Source: CAD feature listing. Evaluate the final solid. Frame: model axes, mm. A direction names the side the tool comes from. Coordinates: 2 decimals unless noted, no trailing zeros. Order: outer loops, then holes, each group sorted by start corner. A loop starts at its lowest first (then second) coordinate and runs counter-clockwise, first axis right, second up. Notation, with made-up numbers: (50.5, 60.25) - (78.5, 60.25) arc R24 cw to (78.5, 95.25) - close; hole circle Ø2 at (-31.5, 67). An arc over 180 degrees is marked (long way). One line per question, with ' | ' between items. Start each with the question number.
(1) Line query: line 1 along X through (y, z) = (7.5, 1.75); line 2 along X through (y, z) = (-4.5, 5.75); line 3 along Y through (x, z) = (-25.5, 6.5). Output: solid intervals per line, ascending.
(2) Contact query for flat-ended pins moving along their axis: P1, Ø4, axis at y = -67.5, z = 9.5, coming from the +X side; P2, Ø1.5, axis at y = -38.5, z = 6, coming from the -X side; P3, Ø1.2, axis at y = 19.5, z = 6.5, coming from the -X side. Output: stop coordinate, or through.
(3) Section B-B (x = -93.5). Return the cut outline in (y, z).
(4) Section C-C (x = -69.5). Return the cut outline in (y, z).
(5) Draft query along X for faces 5 (the flat face through (-25, -92.998, 6)), 6 (the cylindrical face through (73.76, 16.4, 11.01)), 7 (the flat face through (31, -8, 8)). Return one class per face: +X half, -X half, draft (parallel to the pull), parting line (faces both ways), or undercut.
(6) Access query for faces 1 (the flat face through (-90, 20, 6)), 2 (the flat face through (-44.33, -11, 8)), 3 (the flat face through (-72, -2, 6)), 4 (the flat face through (-53, 18.556, 8)). Directions: +Z, -Z, +X, -X, +Y, -Y. A direction counts if a zero-diameter tool reaches every point of the face in a straight line with its end or side. Return the directions, or none.
(7) Section A-A (z = 2). Return the cut outline in (x, y).
from build123d import *

# Parameters (mm, degrees)
BOSS_EXTRUDE1_DEPTH       = 12
SKETCH2_W                 = 25
SKETCH2_H                 = 26.555679241
CUT_EXTRUDE2_DEPTH        = 8
CUT_EXTRUDE8_START        = 4
SKETCH3_W                 = 3
SKETCH3_H                 = 36.555679241
CUT_EXTRUDE8_DEPTH        = 10
SKETCH5_W                 = 12
SKETCH5_H                 = 30.970366581
CUT_EXTRUDE10_DEPTH       = 18
LPATTERN1_COUNT           = 3
LPATTERN1_PITCH           = 42
LPATTERN2_COUNT           = 2
LPATTERN2_PITCH           = 42
CRVPATTERN1_START         = -70.397064899
CRVPATTERN1_OUTLINE_W     = 20.555679241
CRVPATTERN1_OUTLINE_H     = 8
CRVPATTERN1_DEPTH         = 37
CRVPATTERN1_2_DEPTH       = 12
CRVPATTERN1_START_2       = -58.397064899
CRVPATTERN1_3_OUTLINE_W   = 6
CRVPATTERN1_3_OUTLINE_H   = 8
CRVPATTERN1_3_DEPTH       = 25
CRVPATTERN1_START_3       = -53.397064899
CRVPATTERN1_4_OUTLINE_W   = 4
CRVPATTERN1_4_OUTLINE_H   = 8
CRVPATTERN1_4_OUTLINE_W_2 = 6
CRVPATTERN1_4_DEPTH       = 3
FILLET1_R                 = 10
FILLET2_R                 = 10
FILLET3_R                 = 10


# Read off the part's stored shape, not the designer's step: CrvPattern1
with BuildPart() as part:
    # Sketch1 → Boss-Extrude1 (new body)
    with BuildSketch(Plane.XY):
        Polygon((-111.658778955, 20), (77.777911134, 20), (59.936522952, -92.998049549), (-111.658778955, -92.998049549), align=None)
    extrude(amount=BOSS_EXTRUDE1_DEPTH)

    # Sketch2 → Cut-Extrude2 (cut)
    with BuildSketch(Plane.XY.offset(12)):
        with Locations((-6.829680892, 5.27783962)):
            Rectangle(SKETCH2_W, SKETCH2_H)
    cut_extrude2 = extrude(amount=-CUT_EXTRUDE2_DEPTH, mode=Mode.SUBTRACT)

    # Sketch3 → Cut-Extrude8 (cut)
    with BuildSketch(Plane.XY.offset(CUT_EXTRUDE8_START)):
        with Locations((-0.829680892, 4.27783962)):
            Rectangle(SKETCH3_W, SKETCH3_H)
    cut_extrude8 = extrude(amount=CUT_EXTRUDE8_DEPTH, mode=Mode.SUBTRACT)

    # Sketch5 → Cut-Extrude10 (cut)
    with BuildSketch(Plane.XY):
        with Locations((11.670319108, 13.485183291)):
            Rectangle(SKETCH5_W, SKETCH5_H)
    cut_extrude10 = extrude(amount=CUT_EXTRUDE10_DEPTH, mode=Mode.SUBTRACT)

    # LPattern1: Cut-Extrude2, Cut-Extrude8, Cut-Extrude10 ×3
    with Locations(*[(-i * LPATTERN1_PITCH, 0, 0) for i in range(1, LPATTERN1_COUNT)]):
        add(cut_extrude2, mode=Mode.SUBTRACT)
        add(cut_extrude8, mode=Mode.SUBTRACT)
        add(cut_extrude10, mode=Mode.SUBTRACT)

    # LPattern2: Cut-Extrude2, Cut-Extrude8, Cut-Extrude10 ×2
    with Locations(*[(i * LPATTERN2_PITCH, 0, 0) for i in range(1, LPATTERN2_COUNT)]):
        add(cut_extrude2, mode=Mode.SUBTRACT)
        add(cut_extrude8, mode=Mode.SUBTRACT)
        add(cut_extrude10, mode=Mode.SUBTRACT)

    # CrvPattern1 outline → CrvPattern1 (cut)
    with BuildSketch(Plane(origin=(0, 0, 0), x_dir=(0.906467226735628, -0.42227617367573506, 0), z_dir=(0.42227617367573506, 0.9064672267356281, 0)).offset(CRVPATTERN1_START)):
        with Locations((41.40893435, -8)):
            Rectangle(CRVPATTERN1_OUTLINE_W, CRVPATTERN1_OUTLINE_H)
    extrude(amount=CRVPATTERN1_DEPTH, mode=Mode.SUBTRACT)

    # CrvPattern1 2 outline → CrvPattern1 2 (cut)
    with BuildSketch(Plane(origin=(0, 0, 0), x_dir=(0.906467226735628, -0.42227617367573506, 0), z_dir=(0.42227617367573506, 0.9064672267356281, 0)).offset(CRVPATTERN1_START)):
        Polygon((51.68677397, -4), (51.68677397, -12), (62.10146131, -12), (62.10146131, 0), (31.131094729, 0), (31.131094729, -4), align=None)
    extrude(amount=CRVPATTERN1_2_DEPTH, mode=Mode.SUBTRACT)

    # CrvPattern1 3 outline → CrvPattern1 3 (cut)
    with BuildSketch(Plane(origin=(0, 0, 0), x_dir=(0.906467226735628, -0.42227617367573506, 0), z_dir=(0.42227617367573506, 0.9064672267356281, 0)).offset(CRVPATTERN1_START_2)):
        with Locations((28.131094729, -8)):
            Rectangle(CRVPATTERN1_3_OUTLINE_W, CRVPATTERN1_3_OUTLINE_H)
    extrude(amount=CRVPATTERN1_3_DEPTH, mode=Mode.SUBTRACT)

    # CrvPattern1 4 outline → CrvPattern1 4 (cut)
    with BuildSketch(Plane(origin=(0, 0, 0), x_dir=(0.906467226735628, -0.42227617367573506, 0), z_dir=(0.42227617367573506, 0.9064672267356281, 0)).offset(CRVPATTERN1_START_3)):
        with Locations((53.68677397, -8)):
            Rectangle(CRVPATTERN1_4_OUTLINE_W, CRVPATTERN1_4_OUTLINE_H)
        with Locations((22.131094729, -8)):
            Rectangle(CRVPATTERN1_4_OUTLINE_W_2, CRVPATTERN1_4_OUTLINE_H)
    extrude(amount=CRVPATTERN1_4_DEPTH, mode=Mode.SUBTRACT)

    # Fillet1
    fillet1_edges = [part.edges().sort_by_distance(p)[0] for p in [
        (77.777911134, 20, 6),
    ]]
    fillet(fillet1_edges, radius=FILLET1_R)

    # Fillet2
    fillet2_edges = [part.edges().sort_by_distance(p)[0] for p in [
        (-111.658778955, -36.499024774, 0),
        (-111.658778955, 20, 6),
    ]]
    fillet(fillet2_edges, radius=FILLET2_R)

    # Fillet3
    fillet3_edges = [part.edges().sort_by_distance(p)[0] for p in [
        (62.872719189, 20, 0),
        (73.677615847, 16.496310167, 0),
        (67.944638692, -42.278820195, 0),
    ]]
    fillet(fillet3_edges, radius=FILLET3_R)


solid = part.part
Response values:
1) line 1: x = -107.31 to -78.33, -66.33 to -36.33, -24.33 to 5.67, 17.67 to 47.67, 59.67 to 71.4 | line 2: x = -110.71 to -103.33, -78.33 to -61.33, -36.33 to -19.33, 5.67 to 22.67, 47.67 to 72.95 | line 3: y = -93 to -2
2) P1: stops at x = 64.27 | P2: stops at x = -111.12 | P3: stops at x = -106.22
3) outline: (-93, 0) - (20, 0) - (20, 12) - (18.56, 12) - (18.56, 4) - (-8, 4) - (-8, 12) - (-93, 12) - close
4) outline: (-93, 0) - (-2, 0) - (-2, 12) - (-93, 12) - close
5) face 5: draft | face 6: +X half | face 7: undercut
6) face 1: +Z, -Z, +X, -X, +Y | face 2: +Z, +Y | face 3: +Z, -Z, +Y | face 4: +Z
7) outline: (-107.66, -93) - (55.89, -93) - (72, 9.06) arc R6 ccw to (66.08, 16) - (59.67, 16) - (59.67, -2) - (47.67, -2) - (47.67, 20) - (17.67, 20) - (17.67, -2) - (5.67, -2) - (5.67, 20) - (-24.33, 20) - (-24.33, -2) - (-36.33, -2) - (-36.33, 20) - (-66.33, 20) - (-66.33, -2) - (-78.33, -2) - (-78.33, 20) - (-101.66, 20) arc R10 ccw to (-107.66, 18) - close; hole (-1.51, -76.96) - (26.57, -90.04) - (31.63, -79.16) - (3.56, -66.08) - close
